Design review of the part shown in the three views and the two pictorial views. Dimensions are in mm from the part's minimum x, y and z. Round coordinates to 2 decimals unless told otherwise and drop trailing zeros. Write each loop counter-clockwise with the first axis right and the second up, starting at its lowest first coordinate (ties: lowest second). Pieces come first, ordered by that corner, then holes. Notation, with made-up numbers: (50.25, -7) - (98.25, -7) arc R21 cw to (98.25, 6) - close; hole circle Ø7 at (35, -35). An arc over 180 degrees is marked (long way). Use one line per item in the form item = value.
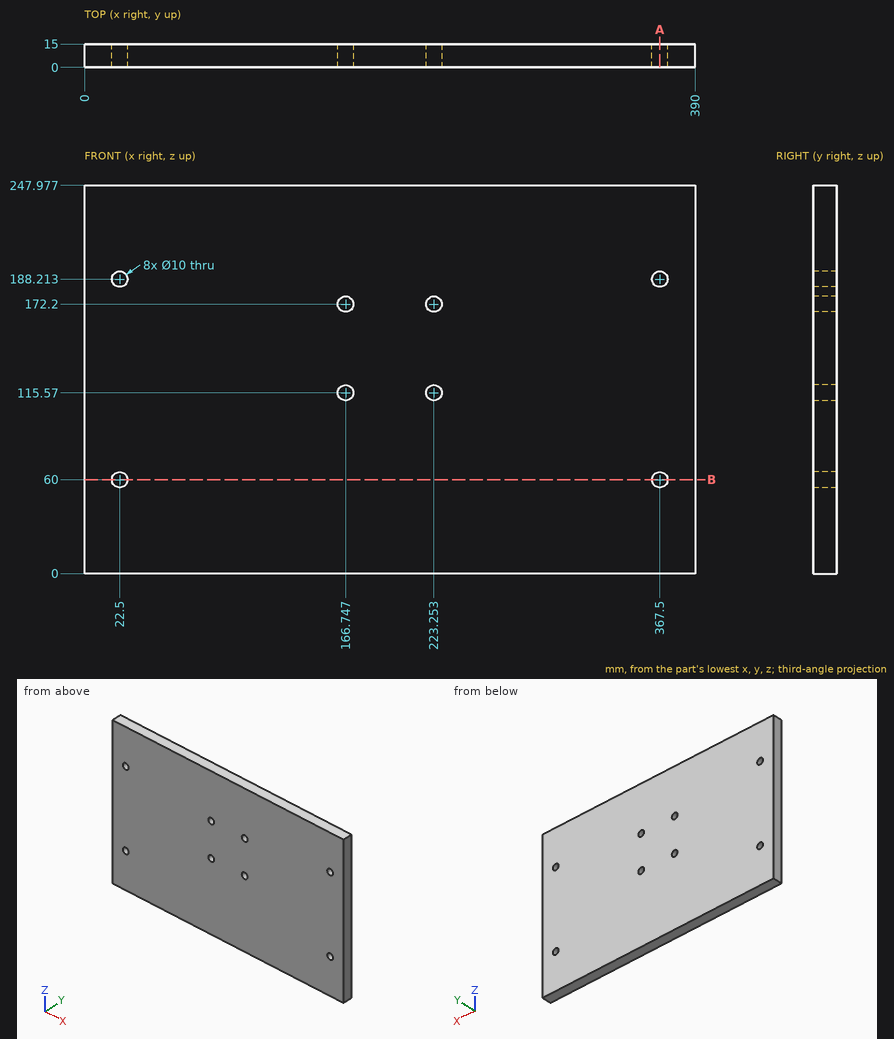
(1) Add section A-A on x = 367.5. Write out the cut boundary in (y, z), then the cut area to 3 significant figures.
Geometry results:
outline = (0, 0) - (15, 0) - (15, 55) - (0, 55) - close; (0, 65) - (15, 65) - (15, 183.21) - (0, 183.21) - close; (0, 193.21) - (15, 193.21) - (15, 247.98) - (0, 247.98) - close
area = 3,420 mm2
(2) Add section B-B on z = 60. Write out the cut boundary in (x, y), then the cut area to 3 significant figures.
Geometry results:
outline = (0, 0) - (17.5, 0) - (17.5, 15) - (0, 15) - close; (27.5, 0) - (362.5, 0) - (362.5, 15) - (27.5, 15) - close; (372.5, 0) - (390, 0) - (390, 15) - (372.5, 15) - close
area = 5,550 mm2
(3) To check wall thickness, follow L1, parallel to Z at x = 22.5, y = 10; L2, parallel to X at y = 3.5, z = 60; L3, parallel to X at y = 10.25, z = 57.5. State the ranges of each line that lie inside material, in increasing order.
Geometry results:
L1 = 0 to 55, 65 to 183.21, 193.21 to 247.98
L2 = 0 to 17.5, 27.5 to 362.5, 372.5 to 390
L3 = 0 to 18.17, 26.83 to 363.17, 371.83 to 390
(4) Insertion check: P1, Ø6, axis at x = 166.75, z = 172.2, coming from the +Y side. The pin has a flat end and moves straight along its axis. Give the tip position at first contact, or say it passes through.
Geometry results:
P1 = through
